CAD build for the part. Positions are in the model's coordinates, mm. Face numbers are marked on the shaded views. A direction names the side the tool comes from. Give positions to 0.01 mm unless a question says otherwise; leave off trailing zeros. Order: outer loops, then holes, each group sorted by start corner. A loop starts at its lowest first (then second) coordinate and runs counter-clockwise, first axis right, second up. Notation, with made-up numbers: M 88.25,42 L 139.25,42 A14 cw 139.25,60 Z; hole C -31,-4.75 d10. An arc over 180 degrees is marked long. Put each result on its own line as item: value. Start each with the question number.
1) Pin check, flat tips, straight feed: pin 1 (2.5 mm diameter, centred on x = 31.9, z = 87.89, fed in from -Y); pin 2 (3 mm diameter, centred on y = -50.5, z = 90.5, fed in from -X); pin 3 (1.8 mm diameter, centred on x = 33.8, y = -46.1, fed in from -Z); pin 4 (4 mm diameter, centred on x = -1, z = 87.5, fed in from +Y). Stop position of each tip, or through.
2) Cut at C-C (x = 2.5). Write the cut outline in (y, z), and give its area (3 significant figures).
3) Drill centre lines: line 1 (X direction, y = -46.1, z = 87.8); line 2 (Z direction, x = 37.05, y = -52.75); line 3 (Z direction, x = 0.5, y = -58.75). Where is each one in solid material? Low to high. Write a range as [from, to].
4) Cut at B-B (z = 85.5). Write the cut outline in (x, y) (3 decimals).
5) Two-plate mould, pull along Z, no slides. Class the marked faces 3, 4, 5 and 6: released by +Z, released by -Z, zero draft, split by the parting line, or undercut.
6) Tool access for the marked faces 1 and 2: list every direction of +Z, -Z, +X, -X, +Y, -Y with a clear straight run to the whole face (end or side of a thin tool).
7) Cut at D-D (y = -61). Write the cut outline in (x, z) (3 decimals), and give its area (3 significant figures).
8) Cut at A-A (x = 42.2). Write the cut outline in (y, z).
```python
from build123d import *

# Parameters (mm, degrees)
PAD011_DEPTH    = 4
PAD012_DEPTH    = 4
PAD012_FACE11_W = 12
PAD012_FACE11_H = 8
PAD013_DEPTH    = 20
PAD014_DEPTH    = 10
SKETCH037_W     = 12
SKETCH037_H     = 2
POCKET014_DEPTH = 5
SKETCH038_W     = 12.9
SKETCH038_H     = 5.9
POCKET015_DEPTH = 5.9
SKETCH039_R     = 1.5
POCKET016_DEPTH = 20
SKETCH040_R     = 1.025
POCKET017_DEPTH = 5
SKETCH041_R     = 1.025
POCKET018_DEPTH = 20
FILLET002_R     = 1


with BuildPart() as part:
    # Sketch035 → Pad011 (new body)
    with BuildSketch(Plane.XY):
        Polygon((-7.5, -57), (19, -57), (19, -51), (24.5, -51), (24.5, -63), (-7.5, -63), align=None)
    extrude(amount=PAD011_DEPTH)

    # Sketch036 (on Face7 of Pad011) → Pad012 (join)
    with BuildSketch(Plane(origin=(0, 0, 0), x_dir=(1, 0, 0), z_dir=(0, 0, -1))):
        Polygon((-7.5, 63), (24.5, 63), (24.5, 51), (17, 51), (17, 55), (-7.5, 55), align=None)
    extrude(amount=PAD012_DEPTH)

    # Pad012 Face11 → Pad013 (add)
    with BuildSketch(Plane(origin=(24.5, -57, 0), x_dir=(0, -1, 0), z_dir=(1, 0, 0))):
        Rectangle(PAD012_FACE11_W, PAD012_FACE11_H)
    extrude(amount=PAD013_DEPTH)

    # Pad013 Face11 → Pad014 (add)
    with BuildSketch(Plane(origin=(31.231132, -51, -0.075472), x_dir=(1, 0, 0), z_dir=(0, 1, 0))):
        Polygon((-12.231132, -0.075472), (-12.231132, -4.075472), (13.268868, -4.075472), (13.268868, 3.924528), (-14.231132, 3.924528), (-14.231132, -0.075472), align=None)
    extrude(amount=PAD014_DEPTH)

    # Sketch037 (on Face9 of Pad014) → Pocket014 (cut)
    with BuildSketch(Plane(origin=(0, 0, -4), x_dir=(1, 0, 0), z_dir=(0, 0, -1))):
        with Locations((0.5, 56)):
            Rectangle(SKETCH037_W, SKETCH037_H)
    extrude(amount=-POCKET014_DEPTH, mode=Mode.SUBTRACT)

    # Sketch038 (on Face10 of Pocket014) → Pocket015 (cut)
    with BuildSketch(Plane(origin=(0, -41, 0), x_dir=(-1, 0, 0), z_dir=(0, 1, 0))):
        with Locations((-37.05, 0.05)):
            Rectangle(SKETCH038_W, SKETCH038_H)
    extrude(amount=-POCKET015_DEPTH, mode=Mode.SUBTRACT)

    # Sketch039 (on Face20 of Pocket015) → Pocket016 (cut)
    with BuildSketch(Plane(origin=(0, -46.9, 0), x_dir=(-1, 0, 0), z_dir=(0, 1, 0))):
        with Locations((-42.2, 0)):
            Circle(SKETCH039_R)
        with Locations((-37.05, 0.05)):
            Circle(SKETCH039_R)
        with Locations((-31.9, 0)):
            Circle(SKETCH039_R)
    extrude(amount=-POCKET016_DEPTH, mode=Mode.SUBTRACT)

    # Sketch040 (on Face8 of Pocket016) → Pocket017 (cut)
    with BuildSketch(Plane(origin=(0, 0, -4), x_dir=(1, 0, 0), z_dir=(0, 0, -1))):
        with Locations((40.3, 46.1)):
            Circle(SKETCH040_R)
        with Locations((33.8, 46.1)):
            Circle(SKETCH040_R)
    extrude(amount=-POCKET017_DEPTH, mode=Mode.SUBTRACT)

    # Sketch041 (on Face19 of Pocket017) → Pocket018 (cut)
    with BuildSketch(Plane.XZ.offset(63)):
        with Locations((0.5, 2.025)):
            Circle(SKETCH041_R)
        with Locations((8.5, 2.025)):
            Circle(SKETCH041_R)
    extrude(amount=-POCKET018_DEPTH, mode=Mode.SUBTRACT)

    # Fillet002
    fillet002_edges = [part.edges().sort_by_distance(p)[0] for p in [
        (18.5, -63, -4),
        (44.5, -63, 0),
        (18.5, -63, 4),
        (-7.5, -63, 0),
        (44.5, -52, -4),
        (0.5, -57, -4),
        (11.75, -55, -4),
        (17, -48, -4),
        (30.75, -41, -4),
        (44.5, -52, 4),
    ]]
    fillet(fillet002_edges, radius=FILLET002_R)


with BuildPart() as part_1:
    # Body002 placement: moved
    add(part.part.moved(Location((0, 0, 87.8927))))


solid = part_1.part
```
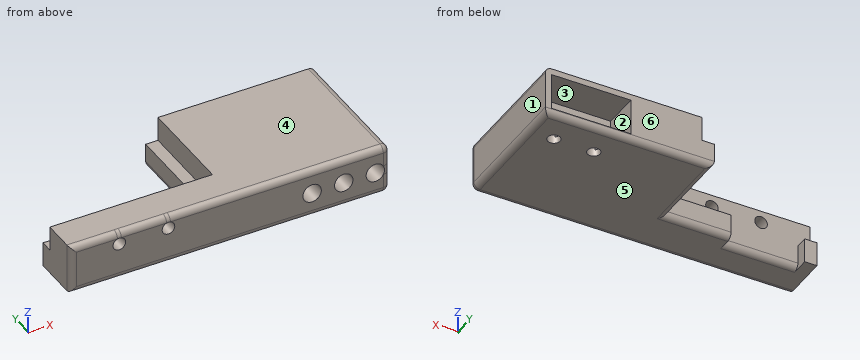
Solution:
1. pin 1: through
1. pin 2: x = 19
1. pin 3: z = 88.89
1. pin 4: y = -57
2. outline: M -63,84.89 A1 ccw -62,83.89 L -58,83.89 A1 ccw -57,84.89 L -57,91.89 L -62,91.89 A1 ccw -63,90.89 Z
2. area: 47.4 mm²
3. line 1: [17, 30.6], [43.5, 44.5]
3. line 2: [83.89, 86.44], [89.44, 91.89]
3. line 3: [83.89, 88.89], [90.94, 91.89]
4. outline: M -7.5,-62 A1 ccw -6.5,-63 L 43.5,-63 A1 ccw 44.5,-62 L 44.5,-41 L 43.5,-41 L 43.5,-46.9 L 40.941,-46.9 A1.025 cw 39.659,-46.9 L 34.441,-46.9 A1.025 cw 33.159,-46.9 L 30.6,-46.9 L 30.6,-41 L 17,-41 L 17,-55 L 6.5,-55 L 6.5,-57 L -5.5,-57 L -5.5,-55 L -7.5,-55 Z
5. face 3: undercut
5. face 4: released by +Z
5. face 5: released by -Z
5. face 6: zero draft
6. face 1: +Z, -Z, +X, +Y, -Y
6. face 2: +Y
7. outline: M -7.5,83.893 L 43.5,83.893 A1 ccw 44.5,84.893 L 44.5,90.893 A1 ccw 43.5,91.893 L -7.5,91.893 Z; hole C 0.5,89.918 d2.05; hole C 8.5,89.918 d2.05; hole C 31.9,87.893 d3; hole C 37.05,87.943 d3; hole C 42.2,87.893 d3
7. area: 388 mm²
8. outline: M -63,84.89 A1 ccw -62,83.89 L -42,83.89 A1 ccw -41,84.89 L -41,84.99 L -46.9,84.99 L -46.9,86.39 L -63,86.39 Z; M -63,89.39 L -46.9,89.39 L -46.9,90.89 L -41,90.89 L -41,91.89 L -62,91.89 A1 ccw -63,90.89 Z
